Could you check a few things on this model? Use its own coordinates, in mm. Coordinates: 2 decimals unless noted, no trailing zeros. Loops run counter-clockwise (first coordinate to the right, second up) from the corner with the lowest first, then second, coordinate; pieces in that order, holes last. Notation, with made-up numbers: (74.25, 51.5) -> (92.25, 51.5) arc R24 cw to (92.25, 69.5) -> close; hole circle Ø3 at (65, 25.5). An arc over 180 degrees is marked (long way). One line per question, with ' | ' between items.
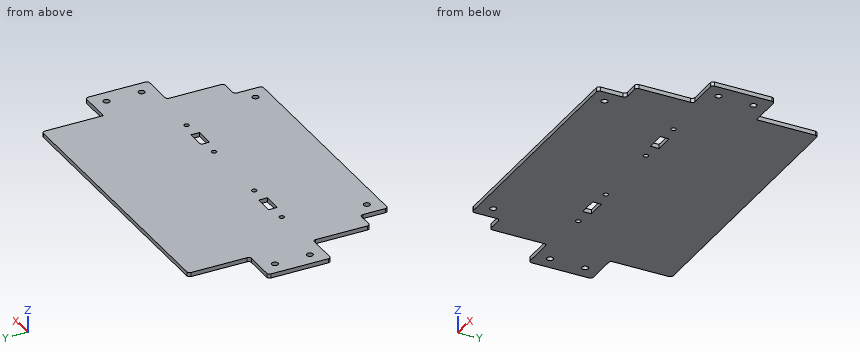
Autodesk Inventor part; units mm, degrees
ref_plane "YZ Plane" through (0, 0, 0) normal (1, 0, 0) x (0, 1, 0)
ref_plane "XZ Plane" through (0, 0, 0) normal (0, 1, 0) x (-1, 0, 0)
ref_plane "XY Plane" through (0, 0, 0) normal (0, 0, 1) x (1, 0, 0)
sketch "Sketch1" plane through (0, 0, 0) normal (0, 0, 1) x (1, 0, 0)
  line L0 (-125, -75) -> (125, -75)
  line L1 (125, -75) -> (125, 75)
  line L2 (125, 75) -> (-125, 75)
  line L3 (-125, 75) -> (-125, -75)
  line L4 (-125, -75) -> (125, 75) construction
  line L5 (125, -75) -> (-125, 75) construction
  point P0 (0, 0)
  dimension "d0" = 150
  dimension "d1" = 250
extrude "Extrusion1" add sketch "Sketch1" along normal blind 3
sketch "Sketch2" plane through (0, 0, 3) normal (0, 0, 1) x (1, 0, 0)
  line L0 (125, -75) -> (125, 75) construction
  line L1 (125, 75) -> (-125, 75) construction
  line L2 (-125, 75) -> (-125, -75) construction
  line L3 (-125, -75) -> (125, -75) construction
  line L4 (-125, 75) -> (-125, -75) construction
  line L5 (125, 75) -> (-125, 75) construction
  line L6 (-125, 75) -> (-100, 75)
  line L7 (-100, 75) -> (-100, 31)
  line L8 (-100, 31) -> (-125, 31)
  line L9 (-125, 31) -> (-125, 75)
  line L10 (-125, -14) -> (-100, -14)
  line L11 (-100, -14) -> (-100, -55)
  line L12 (-100, -55) -> (-86, -55)
  line L13 (-86, -55) -> (-86, -75)
  line L14 (-125, -75) -> (125, -75) construction
  line L15 (-125, -14) -> (-125, -75)
  line L16 (-125, -75) -> (-86, -75)
  line L17 (0, -105) -> (0, 105) construction
  line L18 (125, 75) -> (125, -75) construction
  line L19 (125, 75) -> (125, -75) construction
  line L20 (125, 75) -> (100, 75)
  line L21 (100, 75) -> (100, 31)
  line L22 (100, 31) -> (125, 31)
  line L23 (125, 31) -> (125, 75)
  line L24 (125, -14) -> (100, -14)
  line L25 (100, -14) -> (100, -55)
  line L26 (100, -55) -> (86, -55)
  line L27 (86, -55) -> (86, -75)
  line L28 (125, -14) -> (125, -75)
  line L29 (125, -75) -> (86, -75)
  point P0 (0, 0)
  dimension "d4" = 25
  dimension "d5" = 44
  dimension "d6" = 25
  dimension "d7" = 20
  dimension "d10" = 39
  dimension "d11" = 61
extrude "Extrusion2" cut sketch "Sketch2" against normal blind 3
sketch "Sketch3" plane through (0, 0, 3) normal (0, 0, 1) x (1, 0, 0)
  point P0 (0, 0)
fillet "Fillet1" radius 2 15 edges at (86, -75, 1.5) (86, -55, 1.5) (100, -55, 1.5) (100, -14, 1.5) (125, -14, 1.5) (125, 31, 1.5) (100, 75, 1.5) (-100, 75, 1.5) (-100, 31, 1.5) (-125, 31, 1.5) (-125, -14, 1.5) (-100, -14, 1.5) (-100, -55, 1.5) (-86, -55, 1.5) (-86, -75, 1.5)
sketch "Sketch4" plane through (0, 0, 3) normal (0, 0, 1) x (1, 0, 0)
  circle A0 centre (-115, 21) radius 2.25
  circle A1 centre (-115, -4) radius 2.25
  circle A2 centre (-76, -65) radius 2.25
  line L0 (-125, 29) -> (-125, -12) construction
  line L1 (-102, 31) -> (-123, 31) construction
  line L2 (-123, -14) -> (-102, -14) construction
  line L3 (-86, -57) -> (-86, -73) construction
  line L4 (-84, -75) -> (84, -75) construction
  line L5 (0, -105) -> (0, 105)
  circle A3 centre (115, 21) radius 2.25
  circle A4 centre (115, -4) radius 2.25
  circle A5 centre (76, -65) radius 2.25
  line L6 (125, 29) -> (125, -12) construction
  line L7 (102, 31) -> (123, 31) construction
  line L8 (123, -14) -> (102, -14) construction
  line L9 (86, -57) -> (86, -73) construction
  point P0 (0, 0)
  dimension "d13" = 4.5
  dimension "d14" = 4.5
  dimension "d15" = 4.5
  dimension "d16" = 10
  dimension "d17" = 10
  dimension "d18" = 10
  dimension "d19" = 10
  dimension "d20" = 10
  dimension "d21" = 10
extrude "Extrusion3" cut sketch "Sketch4" against normal blind 3
sketch "Sketch6" plane through (0, 0, 3) normal (0, 0, 1) x (1, 0, 0)
  circle A0 centre (65, -10) radius 1.75
  line L0 (65, -10) -> (27.4, -10) construction
  circle A1 centre (27.4, -10) radius 1.75
  line L1 (-84, -75) -> (84, -75)
  line L2 (100, -53) -> (100, -16)
  line L3 (0, -105.5799) -> (0, 105.5799)
  circle A2 centre (-65, -10) radius 1.75
  line L4 (-65, -10) -> (-27.4, -10) construction
  circle A3 centre (-27.4, -10) radius 1.75
  line L5 (27.4, -10) -> (65, -10) construction
  line L6 (39.4, -13.1) -> (53, -13.1)
  line L7 (53, -13.1) -> (53, -6.9)
  line L8 (53, -6.9) -> (39.4, -6.9)
  line L9 (39.4, -6.9) -> (39.4, -13.1)
  line L10 (39.4, -13.1) -> (53, -6.9) construction
  line L11 (53, -13.1) -> (39.4, -6.9) construction
  line L12 (-39.4, -13.1) -> (-53, -13.1)
  line L13 (-53, -13.1) -> (-53, -6.9)
  line L14 (-53, -6.9) -> (-39.4, -6.9)
  line L15 (-39.4, -6.9) -> (-39.4, -13.1)
  line L16 (-39.4, -13.1) -> (-53, -6.9) construction
  line L17 (-53, -13.1) -> (-39.4, -6.9) construction
  point P0 (0, 0)
  point P1 (46.2, -10)
  point P2 (-46.2, -10)
  dimension "d24" = 3.5
  dimension "d25" = 3.5
  dimension "d26" = 37.6
  dimension "d27" = 65
  dimension "d28" = 35
  dimension "d31" = 13.6
  dimension "d32" = 6.2
  dimension "d33" = 18.8
  dimension "d34" = 18.8
extrude "Extrusion4" cut sketch "Sketch6" against normal blind 10
sketch "Sketch8" plane through (0, 0, 3) normal (0, 0, 1) x (1, 0, 0)
  circle A0 centre (-65, -10) radius 1.75
  circle A1 centre (65, -10) radius 1.75
  line L0 (39.4, -6.9) -> (53, -6.9)
  line L1 (53, -6.9) -> (53, -13.1)
  line L2 (53, -13.1) -> (39.4, -13.1)
  line L3 (39.4, -13.1) -> (39.4, -6.9)
  circle A2 centre (-27.4, -10) radius 1.75
  circle A3 centre (27.4, -10) radius 1.75
  line L4 (-39.4, -13.1) -> (-53, -13.1)
  line L5 (-53, -13.1) -> (-53, -6.9)
  line L6 (-53, -6.9) -> (-39.4, -6.9)
  line L7 (-39.4, -6.9) -> (-39.4, -13.1)
  circle A4 centre (-76, -65) radius 2.25
  circle A5 centre (115, 21) radius 2.25
  circle A6 centre (-115, -4) radius 2.25
  circle A7 centre (76, -65) radius 2.25
  circle A8 centre (115, -4) radius 2.25
  circle A9 centre (-115, 21) radius 2.25
  arc A10 (-86, -73) -> (-84, -75) centre (-84, -73) ccw
  line L8 (-84, -75) -> (84, -75)
  arc A11 (84, -75) -> (86, -73) centre (84, -73) ccw
  line L9 (86, -73) -> (86, -57)
  arc A12 (88, -55) -> (86, -57) centre (88, -57) ccw
  line L10 (88, -55) -> (98, -55)
  arc A13 (98, -55) -> (100, -53) centre (98, -53) ccw
  line L11 (100, -53) -> (100, -16)
  arc A14 (102, -14) -> (100, -16) centre (102, -16) ccw
  line L12 (102, -14) -> (123, -14)
  arc A15 (123, -14) -> (125, -12) centre (123, -12) ccw
  line L13 (125, -12) -> (125, 29)
  arc A16 (125, 29) -> (123, 31) centre (123, 29) ccw
  line L14 (123, 31) -> (100, 31)
  line L15 (100, 31) -> (100, 73)
  arc A17 (100, 73) -> (98, 75) centre (98, 73) ccw
  line L16 (98, 75) -> (-98, 75)
  arc A18 (-98, 75) -> (-100, 73) centre (-98, 73) ccw
  line L17 (-100, 73) -> (-100, 33)
  arc A19 (-102, 31) -> (-100, 33) centre (-102, 33) ccw
  line L18 (-102, 31) -> (-123, 31)
  arc A20 (-123, 31) -> (-125, 29) centre (-123, 29) ccw
  line L19 (-125, 29) -> (-125, -12)
  arc A21 (-125, -12) -> (-123, -14) centre (-123, -12) ccw
  line L20 (-123, -14) -> (-102, -14)
  arc A22 (-100, -16) -> (-102, -14) centre (-102, -16) ccw
  line L21 (-100, -16) -> (-100, -53)
  arc A23 (-100, -53) -> (-98, -55) centre (-98, -53) ccw
  line L22 (-98, -55) -> (-88, -55)
  arc A24 (-86, -57) -> (-88, -55) centre (-88, -57) ccw
  line L23 (-86, -57) -> (-86, -73)
  point P0 (0, 0)
equation "\"d6\" = d4"
equation "\"d14\" = d13"
equation "\"d15\" = d14"
equation "\"d17\" = d16"
equation "\"d18\" = d16"
equation "\"d19\" = d16"
equation "\"d20\" = d19"
equation "\"d21\" = d19"
equation "\"d25\" = d24"
properties part number "BackAcrylicSheet"
Q1. For pin 1 (0.9 mm diameter, centred on y = -32.5, z = 2, fed in from -X); pin 2 (0.9 mm diameter, centred on x = 114, z = 1.5, fed in from -Y), each with a flat end and sliding along its axis, tell me the tip position at first contact or that it passes through.
Values follow:
pin 1: stops at x = -100 | pin 2: stops at y = -14
Q2. Please list where these lines run through material, in increasing order: L1, parallel to Y at x = -115, z = 0.7; L2, parallel to Y at x = -65, z = 1.45; L3, parallel to Y at x = -44.5, z = 1.15. Write a range as [from, to].
Values follow:
L1: y = [-14, -6.25], [-1.75, 18.75], [23.25, 31] | L2: y = [-75, -11.75], [-8.25, 75] | L3: y = [-75, -13.1], [-6.9, 75]
Q3. Imagine slicing it at C-C on z = 1.1. Give the number of separate pieces and of enclosed holes in the cut face, plus the area to 3 significant figures.
Values follow:
separate pieces: 1 | enclosed holes: 12 | area: 31,400 mm2
Q4. Imagine slicing it at A-A on y = 56. Write out the boundary of the cut face in (x, z), plus the area to 3 significant figures.
Values follow:
outline: (-100, 0) -> (100, 0) -> (100, 3) -> (-100, 3) -> close | area: 600 mm2
Q5. Imagine slicing it at B-B on x = -106.5. Write out the boundary of the cut face in (y, z), plus the area to 3 significant figures.
Values follow:
outline: (-14, 0) -> (31, 0) -> (31, 3) -> (-14, 3) -> close | area: 135 mm2
